```python
from build123d import *

# Parameters (mm, degrees)
BOSS_EXTRUDE1_DEPTH = 7.9
SKETCH2_R           = 3.144549921
BOSS_EXTRUDE3_DEPTH = 0.5
SKETCH3_R           = 2.455888386
BOSS_EXTRUDE4_DEPTH = 7.9
SKETCH4_R           = 2.65462565
BOSS_EXTRUDE5_DEPTH = 0.3
SKETCH5_R           = 2.198604039
CUT_EXTRUDE1_DEPTH  = 7.9
CUT_EXTRUDE2_DEPTH  = 3.3
FILLET1_R           = 0.3
CUT_EXTRUDE5_START  = 9
SKETCH7_R           = 3.144549921
CUT_EXTRUDE5_DEPTH  = 9
SKETCH8_R           = 1.75
BOSS_EXTRUDE6_DEPTH = 3


with BuildPart() as part:
    # Sketch1 → Boss-Extrude1 (new body)
    with BuildSketch(Plane.XY):
        Polygon((-2.4, 0.895), (-2.4, 0), (0, 0), (0, 2.4), (-0.9, 2.4), (-0.9, 0.895), align=None)
        Polygon((0, 0), (-2.4, 0), (-2.4, -0.895), (-0.9, -0.895), (-0.9, -2.4), (0, -2.4), align=None)
        Polygon((0, 2.4), (0, 0), (2.4, 0), (2.4, 0.895), (0.9, 0.895), (0.9, 2.4), align=None)
        Polygon((2.4, 0), (0, 0), (0, -2.4), (0.9, -2.4), (0.9, -0.895), (2.4, -0.895), align=None)
    extrude(amount=BOSS_EXTRUDE1_DEPTH)

    # Sketch2 → Boss-Extrude3 (add)
    with BuildSketch(Plane(origin=(0, 0, 0), x_dir=(-1, 0, 0), z_dir=(0, 0, -1))):
        Circle(SKETCH2_R)
    extrude(amount=BOSS_EXTRUDE3_DEPTH)

    # Sketch3 → Boss-Extrude4 (add)
    with BuildSketch(Plane(origin=(0, 0, -0.5), x_dir=(-1, 0, 0), z_dir=(0, 0, -1))):
        Circle(SKETCH3_R)
    extrude(amount=BOSS_EXTRUDE4_DEPTH)

    # Sketch4 → Boss-Extrude5 (add)
    with BuildSketch(Plane(origin=(0, 0, -8.4), x_dir=(-1, 0, 0), z_dir=(0, 0, -1))):
        Circle(SKETCH4_R)
    extrude(amount=-BOSS_EXTRUDE5_DEPTH)

    # Sketch5 → Cut-Extrude1 (cut)
    with BuildSketch(Plane(origin=(0, 0, -8.4), x_dir=(-1, 0, 0), z_dir=(0, 0, -1))):
        Circle(SKETCH5_R)
    extrude(amount=-CUT_EXTRUDE1_DEPTH, mode=Mode.SUBTRACT)

    # Sketch6 → Cut-Extrude2 (cut)
    with BuildSketch(Plane(origin=(0, 0, -8.4), x_dir=(-1, 0, 0), z_dir=(0, 0, -1))):
        with BuildLine():
            Line((0.375484044, 2.166303638), (0.375484044, 2.627936276))
            ThreePointArc((0.375484044, 2.627936276), (0.188215694, 2.6479449), (0, 2.65462565))
            Line((0, 2.65462565), (0, 2.198604039))
            ThreePointArc((0, 2.198604039), (0.188435389, 2.190514055), (0.375484044, 2.166303638))
        make_face()
        with BuildLine():
            Line((0, 2.198604039), (0, 2.65462565))
            ThreePointArc((0, 2.65462565), (-0.188215694, 2.6479449), (-0.375484044, 2.627936276))
            Line((-0.375484044, 2.627936276), (-0.375484044, 2.166303638))
            ThreePointArc((-0.375484044, 2.166303638), (-0.188435389, 2.190514055), (0, 2.198604039))
        make_face()
        with BuildLine():
            ThreePointArc((0, -2.65462565), (0.188215694, -2.6479449), (0.375484044, -2.627936276))
            Line((0.375484044, -2.627936276), (0.375484044, -2.166303638))
            ThreePointArc((0.375484044, -2.166303638), (0, -2.198604039), (-0.375484044, -2.166303638))
            Line((-0.375484044, -2.166303638), (-0.375484044, -2.627936276))
            ThreePointArc((-0.375484044, -2.627936276), (-0.188215694, -2.6479449), (0, -2.65462565))
        make_face()
    extrude(amount=-CUT_EXTRUDE2_DEPTH, mode=Mode.SUBTRACT)

    # Fillet1
    fillet1_edges = [part.edges().sort_by_distance(p)[0] for p in [
        (0.375484044, 2.296659081, -5.1),
        (-0.375484044, 2.296659081, -5.1),
        (-0.375484044, -2.296659081, -5.1),
        (0.375484044, -2.296659081, -5.1),
    ]]
    fillet(fillet1_edges, radius=FILLET1_R)

    # Sketch7 → Cut-Extrude5 (cut)
    with BuildSketch(Plane.XY.offset(CUT_EXTRUDE5_START)):
        with Locations(Location((0, 0, 0), (0, 0, 180))):
            Circle(SKETCH7_R)
    extrude(amount=-CUT_EXTRUDE5_DEPTH, mode=Mode.SUBTRACT)

    # Sketch8 → Boss-Extrude6 (add)
    with BuildSketch(Plane.XY):
        Circle(SKETCH8_R)
    extrude(amount=BOSS_EXTRUDE6_DEPTH)

    # Sketch9 → Revolve1 (revolve)
    with BuildSketch(Plane(origin=(0, 0, 0), x_dir=(0, 0, -1), z_dir=(1, 0, 0))):
        with BuildLine():
            Line((-5.297920188, 3.009117544), (-5.297920188, -2.990882456))
            ThreePointArc((-5.297920188, -2.990882456), (-2.297920188, 0.009117544), (-5.297920188, 3.009117544))
        make_face()
    revolve(axis=Axis((0, 3.009117544, 5.297920188), (0, -1, 0)))


solid = part.part
```
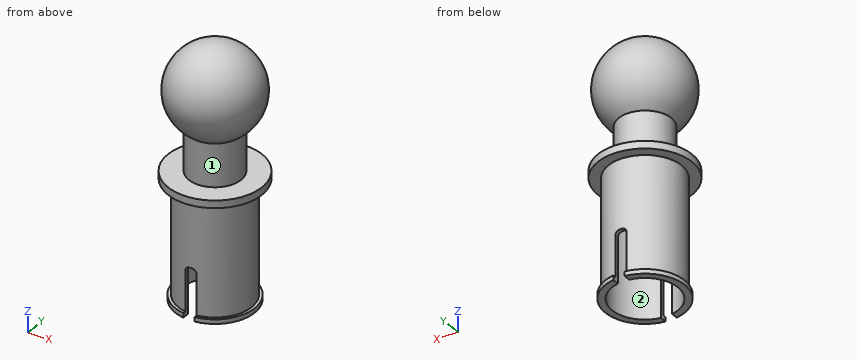
Geometry check sheet. Reference: the model listing, model coordinates, mm. Face numbers are marked on the shaded views. Coordinates: 2 decimals unless noted, no trailing zeros. Write each loop counter-clockwise with the first axis right and the second up, starting at its lowest first coordinate (ties: lowest second). Pieces come first, ordered by that corner, then holes. Notation, with made-up numbers: (-6, 70.25) -> (38, 70.25) arc R18 cw to (38, 81.25) -> close; hole circle Ø5 at (57.25, 69). An arc over 180 degrees is marked (long way). Use CSV: the item, a comma, the result in double quotes. Start each with the question number.
Item 1: Cross-section at D-D, the plane z = -2.75. Record the cut outline in (x, y), plus the area to 3 significant figures.
Item 2: Cross-section at C-C, the plane x = 1.5. Record the cut outline in (y, z).
Item 3: Cross-section at A-A, the plane y = 1.25. Record the cut outline in (x, z), plus the area to 3 significant figures.
Item 4: Thickness scan on line 1 (Y direction, x = 0, z = -3.75); line 2 (Z direction, x = 2.5, y = -0.25); line 3 (Z direction, x = -0.75, y = -3). Record the ranges inside material, lowest first.
Item 5: Mould release check, pull along Z, two halves, no side actions. Record for the marked faces 1 and 2: released by +Z, released by -Z, zero draft, split by the parting line, or undercut.
Item 6: Depth check by flat-ended pin: pin 1 Ø3 at (x, y) = (-0.5, -1.5) entering from -Z; pin 2 Ø0.5 at (y, z) = (-2.5, -7) entering from -X; pin 3 Ø1.9 at (x, y) = (0.5, -1.5) entering from +Z; pin 4 Ø1.3 at (x, y) = (0, 0.5) entering from -Z. Enter the tip coordinate at first touch or a pass-through.
Item 7: Cross-section at B-B, the plane z = 2. Record the cut outline in (x, y).
Answers:
1,outline,"circle Ø4.91 at (0, 0); hole circle Ø4.4 at (0, 0)"
1,area,"3.76 mm^2"
2,outline,"(-2.76, -0.5) -> (-1.94, -0.5) -> (-1.94, -8.1) -> (-2.19, -8.1) -> (-2.19, -8.4) -> (-1.61, -8.4) -> (-1.61, -0.5) -> (1.61, -0.5) -> (1.61, -8.4) -> (2.19, -8.4) -> (2.19, -8.1) -> (1.94, -8.1) -> (1.94, -0.5) -> (2.76, -0.5) -> (2.76, 0) -> (0.9, 0) -> (0.9, 2.86) arc R2.6 ccw (long way) to (-0.9, 2.86) -> (-0.9, 0) -> (-2.76, 0) -> close"
3,outline,"(-2.89, -0.5) -> (-2.11, -0.5) -> (-2.11, -8.1) -> (-2.34, -8.1) -> (-2.34, -8.4) -> (-1.81, -8.4) -> (-1.81, -0.5) -> (1.81, -0.5) -> (1.81, -8.4) -> (2.34, -8.4) -> (2.34, -8.1) -> (2.11, -8.1) -> (2.11, -0.5) -> (2.89, -0.5) -> (2.89, 0) -> (1.22, 0) -> (1.22, 2.86) arc R2.73 ccw (long way) to (-1.22, 2.86) -> (-1.22, 0) -> (-2.89, 0) -> close"
3,area,"37.8 mm^2"
4,line 1,"-2.46 to -2.2, 2.2 to 2.46"
4,line 2,"-8.4 to -8.1, -0.5 to 0, 3.66 to 6.94"
4,line 3,"-0.5 to 0"
5,face 1,"undercut"
5,face 2,"zero draft"
6,pin 1,"z = -8.4"
6,pin 2,"x = -0.98"
6,pin 3,"z = 8.23"
6,pin 4,"z = -0.5"
7,outline,"circle Ø3.5 at (0, 0)"
